Input: dimensioned drawing with shaded views. Units: mm. Origin: part minimum x, y, z. Coordinates: 2 decimals unless noted, no trailing zeros. Order: outer loops, then holes, each group sorted by start corner. A loop starts at its lowest first (then second) coordinate and runs counter-clockwise, first axis right, second up. Notation, with made-up numbers: (6, 9.25) - (51, 9.25) arc R21 cw to (51, 37.25) - close; hole circle Ø6 at (65.5, 40). An arc over 180 degrees is marked (long way). One line per question, with ' | ' between items. Start each with the question number.
(1) Section B-B (x = 11). Return the cut outline in (y, z).
(2) Section C-C (x = 78). Return the cut outline in (y, z), then the cut area to 3 significant figures.
(3) Contact query for a flat-ended pin moving along its axis: P1, Ø3.5, axis at x = 21.803, y = 7.365, coming from the +Z side. Output: stop coordinate, or through.
(4) Section A-A (z = 0.7). Return the cut outline in (x, y) (3 decimals), then the cut area to 3 significant figures.
(5) Line query: line 1 along X through (y, z) = (6.5, 0.3); line 2 along X through (y, z) = (14.25, 1.55); line 3 along X through (y, z) = (5.5, 0.25). Output: solid intervals per line, ascending.
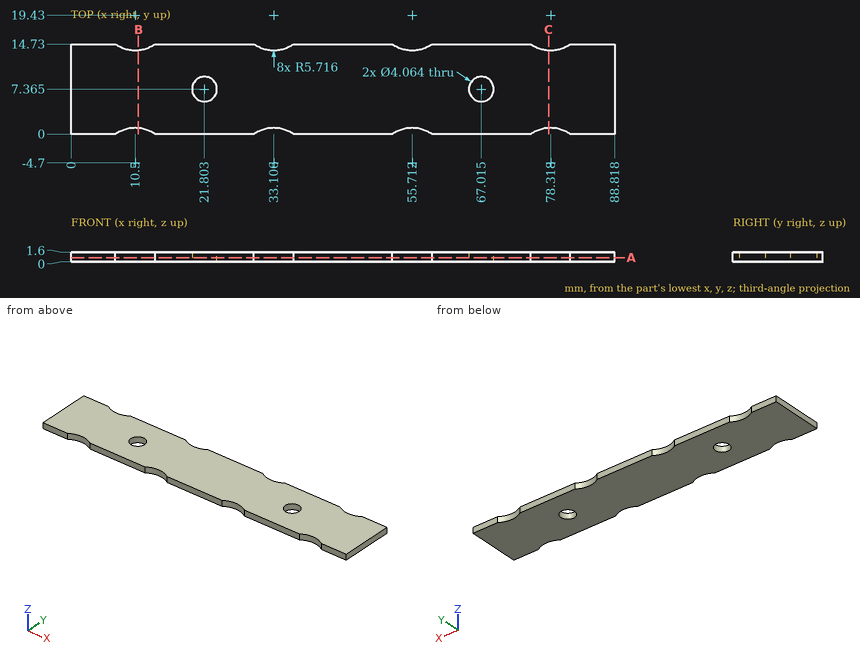
Response values:
1) outline: (0.99, 0) - (13.74, 0) - (13.74, 1.6) - (0.99, 1.6) - close
2) outline: (1.01, 0) - (13.72, 0) - (13.72, 1.6) - (1.01, 1.6) - close | area: 20.3 mm²
3) P1: passes through
4) outline: (0, 0) - (7.247, 0) arc R5.716 cw to (13.753, 0) - (29.853, 0) arc R5.716 cw to (36.359, 0) - (52.459, 0) arc R5.716 cw to (58.965, 0) - (75.065, 0) arc R5.716 cw to (81.571, 0) - (88.818, 0) - (88.818, 14.73) - (81.571, 14.73) arc R5.716 cw to (75.065, 14.73) - (58.965, 14.73) arc R5.716 cw to (52.459, 14.73) - (36.359, 14.73) arc R5.716 cw to (29.853, 14.73) - (13.753, 14.73) arc R5.716 cw to (7.247, 14.73) - (0, 14.73) - close; hole circle Ø4.064 at (21.803, 7.365); hole circle Ø4.064 at (67.015, 7.365) | area: 1,250 mm²
5) line 1: x = 0 to 19.96, 23.64 to 65.18, 68.85 to 88.82 | line 2: x = 0 to 8.08, 12.92 to 30.69, 35.52 to 53.3, 58.13 to 75.9, 80.73 to 88.82 | line 3: x = 0 to 21, 22.61 to 66.21, 67.82 to 88.82
